from build123d import *

# Parameters (mm, degrees)
SKETCH1_W           = 120
SKETCH1_H           = 120
BOSS_EXTRUDE1_DEPTH = 90
FILLET1_R           = 10
SHELL1_T            = -4


with BuildPart() as part:
    # Sketch1 → Boss-Extrude1 (new body)
    with BuildSketch(Plane.XY):
        with Locations((60, 60)):
            Rectangle(SKETCH1_W, SKETCH1_H)
    extrude(amount=BOSS_EXTRUDE1_DEPTH)

    # Fillet1
    fillet1_edges = [part.edges().sort_by_distance(p)[0] for p in [
        (0, 120, 45),
        (120, 120, 45),
        (120, 0, 45),
        (0, 0, 45),
    ]]
    fillet(fillet1_edges, radius=FILLET1_R)

    # Shell1
    shell1_openings = [part.faces().sort_by_distance(p)[0] for p in [
        (60, 60, 90),
    ]]
    offset(amount=SHELL1_T, openings=shell1_openings, kind=Kind.INTERSECTION)


solid = part.part
Geometry check sheet. Reference: the model listing, model coordinates, mm. A direction names the side the tool comes from. Round coordinates to 2 decimals unless told otherwise and drop trailing zeros. Loops run counter-clockwise (first coordinate to the right, second up) from the corner with the lowest first, then second, coordinate; pieces in that order, holes last. Notation, with made-up numbers: (-30.5, 42) - (-3.5, 42) arc R21 cw to (-3.5, 78) - close; hole circle Ø7 at (42.5, 52.25). An arc over 180 degrees is marked (long way). One line per question, with ' | ' between items. Start each with the question number.
1. Cross-section at A-A on x = 83. Record the cut outline in (y, z).
2. Cross-section at B-B on z = 31. Record the cut outline in (x, y), then the cut area to 3 significant figures.
3. Depth check by flat-ended pin: pin 1 (10 mm diameter, centred on x = 21.5, y = 48, fed in from +Z). Enter the tip coordinate at first touch or a pass-through.
4. Draft check along Y on faces 3 (the face through (59, 120, 44)), 4 (the face through (116.99, 2.85, 45.63)), 5 (the face through (5.711, 114.196, 47.602)). Enter one of: released by +Y, released by -Y, zero draft, split by the parting line, or undercut.
5. Scan lines: line 1 (X direction, y = 67, z = 70.5); line 2 (Z direction, x = 109.5, y = 22.5). Record each from-to range of solid material in increasing order. Write a range as [from, to].
6. Tool access check on faces 1 (the face through (116, 59, 46)), 2 (the face through (0, 59, 44)). Record the directions out of +Z, -Z, +X, -X, +Y, -Y that give a thin tool (end or side, any length) a straight path to the whole face; none if there is none.
Taken from the geometry:
1) outline: (0, 0) - (120, 0) - (120, 90) - (116, 90) - (116, 4) - (4, 4) - (4, 90) - (0, 90) - close
2) outline: (0, 10) arc R10 ccw to (10, 0) - (110, 0) arc R10 ccw to (120, 10) - (120, 110) arc R10 ccw to (110, 120) - (10, 120) arc R10 ccw to (0, 110) - close; hole (4, 10) arc R6 ccw to (10, 4) - (110, 4) arc R6 ccw to (116, 10) - (116, 110) arc R6 ccw to (110, 116) - (10, 116) arc R6 ccw to (4, 110) - close | area: 1,800 mm²
3) pin 1: z = 4
4) face 3: released by +Y | face 4: released by -Y | face 5: undercut
5) line 1: [0, 4], [116, 120] | line 2: [0, 4]
6) face 1: +Z | face 2: +Z, -Z, -X, +Y, -Y
